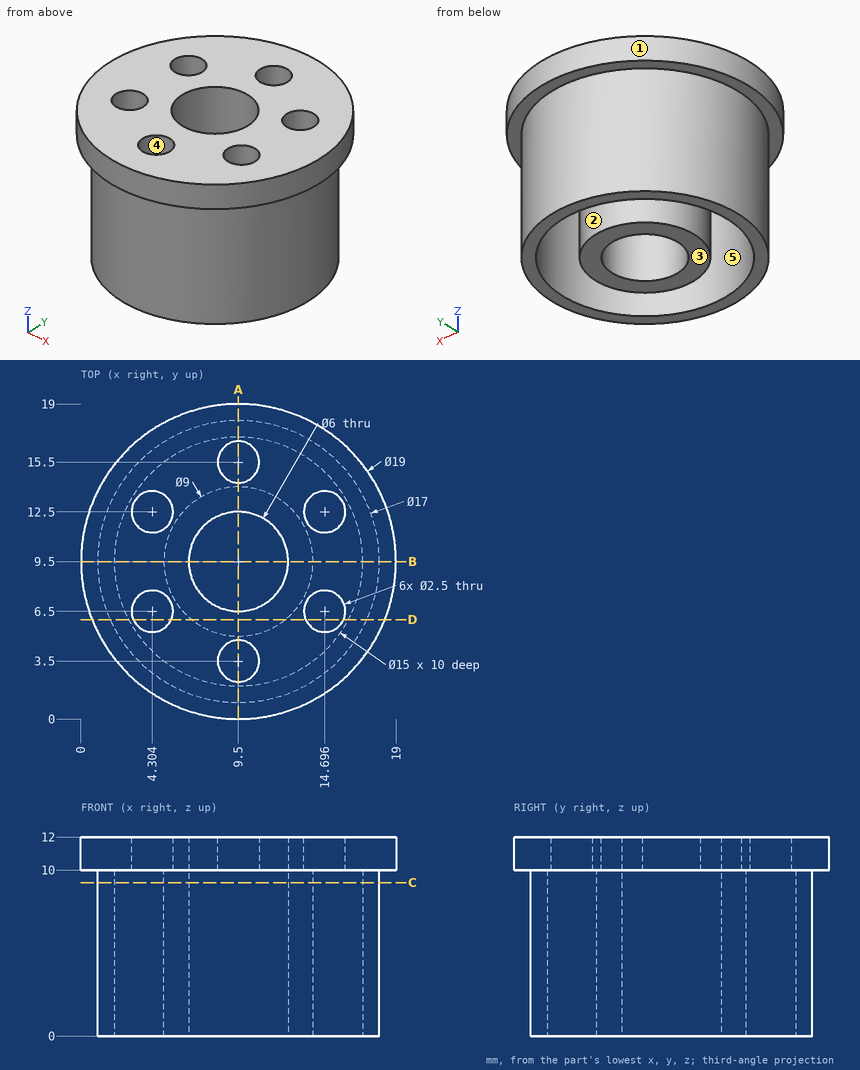
Study the drawing (mm; zero at the part's minimum x, y, z) and answer. A direction names the side the tool comes from. Round coordinates to 2 decimals unless told otherwise and drop trailing zeros. Loops run counter-clockwise (first coordinate to the right, second up) from the corner with the lowest first, then second, coordinate; pieces in that order, holes last.
Q1. Section B-B, the plane y = 9.5 is taken. Determine the outline of the cut face in (x, z), then the cut area to 3 significant figures.
Q2. Section C-C, the plane z = 9.25 is taken. Determine the outline of the cut face in (x, y).
Q3. Given pin 1 Ø1 at (y, z) = (15.5, 3) entering from +X; pin 2 Ø1.5 at (x, z) = (3.5, 9.5) entering from -Y; pin 3 Ø3 at (y, z) = (6, 6.5) entering from -X, each flat-ended and moving along its own axis, determine where each tip first touches the part or whether it passes through.
Q4. Section D-D, the plane y = 6 is taken. Determine the outline of the cut face in (x, z).
Q5. Which of the six approach directions +Z, -Z, +X, -X, +Y, -Y give full straight-line access (tool end or side, diameter ignored) to the marked faces 4 and 5?
Q6. For a pull along Y with two mould halves and no side action, classify the marked faces 1, 2 and 3 as released by +Y, released by -Y, zero draft, split by the parting line, or undercut.
Q7. Find the intervals of material crossed by line 1 (Y direction, x = 9.5, z = 5); line 2 (Y direction, x = 12, z = 3.5) (1 decimal); line 3 (Y direction, x = 6, z = 2) (1 decimal), in increasing order.
Q8. Section A-A, the plane x = 9.5 is taken. Determine the outline of the cut face in (y, z), then the cut area to 3 significant figures.
Completed:
1. outline: (0, 10) - (1, 10) - (1, 0) - (2, 0) - (2, 10) - (5, 10) - (5, 0) - (6.5, 0) - (6.5, 12) - (0, 12) - close; (12.5, 0) - (14, 0) - (14, 10) - (17, 10) - (17, 0) - (18, 0) - (18, 10) - (19, 10) - (19, 12) - (12.5, 12) - close
1. area: 76.0 mm2
2. outline: circle Ø17 at (9.5, 9.5); circle Ø9 at (9.5, 9.5); hole circle Ø15 at (9.5, 9.5); hole circle Ø6 at (9.5, 9.5)
3. pin 1: stops at x = 15.98
3. pin 2: stops at y = 1.71
3. pin 3: stops at x = 1.24
4. outline: (0.67, 10) - (1.75, 10) - (1.75, 0) - (2.87, 0) - (2.87, 10) - (3.16, 10) - (3.16, 12) - (0.67, 12) - close; (5.45, 10) - (6.67, 10) - (6.67, 0) - (12.33, 0) - (12.33, 10) - (13.55, 10) - (13.55, 12) - (5.45, 12) - close; (15.84, 10) - (16.13, 10) - (16.13, 0) - (17.25, 0) - (17.25, 10) - (18.33, 10) - (18.33, 12) - (15.84, 12) - close
5. face 4: +Z, -Z
5. face 5: -Z
6. face 1: split by the parting line
6. face 2: undercut
6. face 3: zero draft
7. line 1: y = 1 to 2, 5 to 6.5, 12.5 to 14, 17 to 18
7. line 2: y = 1.4 to 2.4, 5.8 to 7.8, 11.2 to 13.2, 16.6 to 17.6
7. line 3: y = 1.8 to 2.9, 6.7 to 12.3, 16.1 to 17.2
8. outline: (0, 10) - (1, 10) - (1, 0) - (2, 0) - (2, 10) - (2.25, 10) - (2.25, 12) - (0, 12) - close; (4.75, 10) - (5, 10) - (5, 0) - (6.5, 0) - (6.5, 12) - (4.75, 12) - close; (12.5, 0) - (14, 0) - (14, 10) - (14.25, 10) - (14.25, 12) - (12.5, 12) - close; (16.75, 10) - (17, 10) - (17, 0) - (18, 0) - (18, 10) - (19, 10) - (19, 12) - (16.75, 12) - close
8. area: 66.0 mm2
